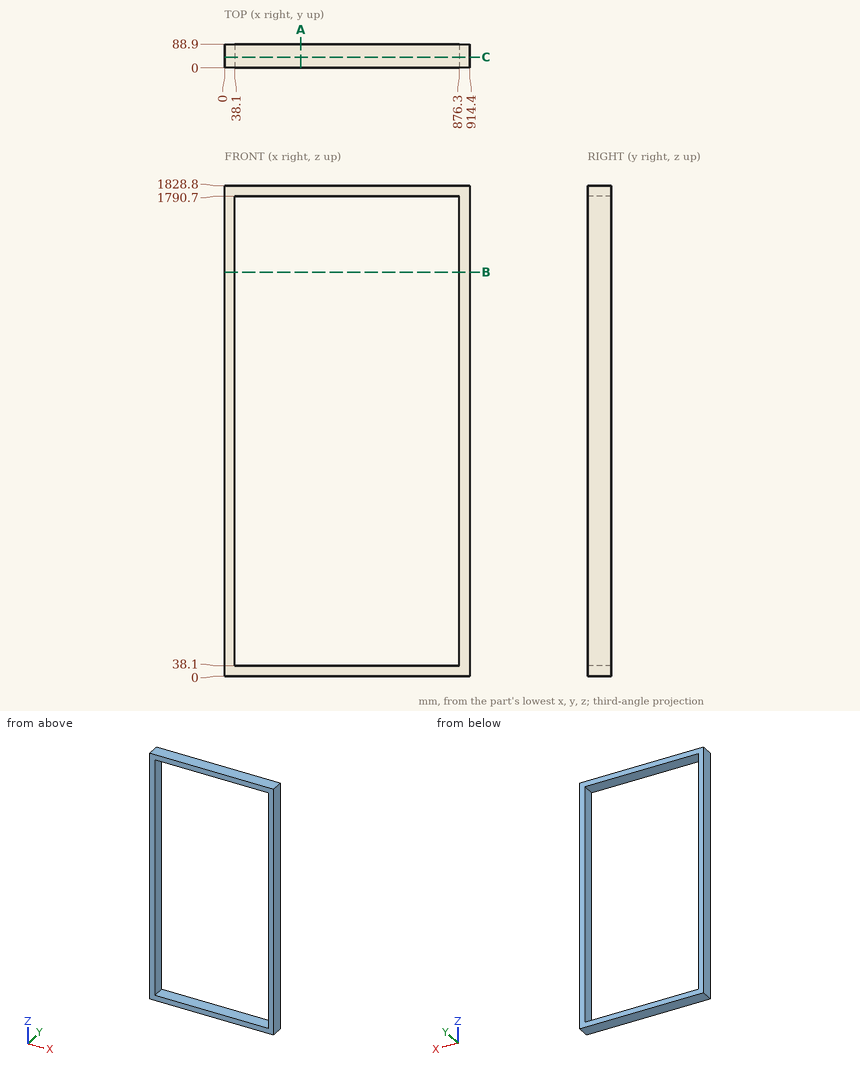
Study the drawing (mm; zero at the part's minimum x, y, z) and answer. Coordinates: 2 decimals unless noted, no trailing zeros. Write each loop counter-clockwise with the first axis right and the second up, starting at its lowest first coordinate (ties: lowest second). Pieces come first, ordered by that corner, then holes. Notation, with made-up numbers: (79, 18) - (127, 18) arc R13 cw to (127, 42) - close; hole circle Ø5 at (81, -20.75). An arc over 180 degrees is marked (long way). Return JSON: item names as keys, results as strings. Group by question number.
1. A cutting plane is placed at A-A, the plane x = 285. Determine the outline of the cut face in (y, z).
2. Straight lines are drawn through the part: L1, parallel to X at y = 61.5, z = 1199; L2, parallel to Z at x = 302.5, y = 24.5. For each, find the intervals that lie inside material, in ascending order.
3. A cutting plane is placed at C-C, the plane y = 40. Determine the outline of the cut face in (x, z).
4. A cutting plane is placed at B-B, the plane z = 1507. Determine the outline of the cut face in (x, y).
Ans:
{
 "1": {"outline": "(0, 0) - (88.9, 0) - (88.9, 38.1) - (0, 38.1) - close; (0, 1790.7) - (88.9, 1790.7) - (88.9, 1828.8) - (0, 1828.8) - close"},
 "2": {"L1": "0 to 38.1, 876.3 to 914.4", "L2": "0 to 38.1, 1790.7 to 1828.8"},
 "3": {"outline": "(0, 0) - (914.4, 0) - (914.4, 1828.8) - (0, 1828.8) - close; hole (38.1, 38.1) - (876.3, 38.1) - (876.3, 1790.7) - (38.1, 1790.7) - close"},
 "4": {"outline": "(0, 0) - (38.1, 0) - (38.1, 88.9) - (0, 88.9) - close; (876.3, 0) - (914.4, 0) - (914.4, 88.9) - (876.3, 88.9) - close"}
}
